CAD build for the part. Positions are in the model's coordinates, mm. Face numbers are marked on the shaded views. A direction names the side the tool comes from. Round coordinates to 2 decimals unless told otherwise and drop trailing zeros. Loops run counter-clockwise (first coordinate to the right, second up) from the corner with the lowest first, then second, coordinate; pieces in that order, holes last.
from build123d import *

# Parameters (mm, degrees)
SKETCH_1_R          = 3.1
EXTRUDE_1_DEPTH     = 5.7
SKETCH_2_R          = 2
EXTRUDE_2_DEPTH     = 7
SKETCH_3_R          = 1.25
EXTRUDE_3_DEPTH     = 6
CHAMFER_1_SIZE      = 0.2535
CHAMFER_2_SIZE      = 0.5
SKETCH_5_W          = 1.1
SKETCH_5_H          = 7
CUT_EXTRUDE_1_DEPTH = 1.2


with BuildPart() as part:
    # Эскиз1 → Бобышка-Вытянуть1 (new body)
    with BuildSketch(Plane.XY):
        Circle(SKETCH_1_R)
    extrude(amount=EXTRUDE_1_DEPTH)

    # Эскиз2 → Бобышка-Вытянуть2 (add)
    with BuildSketch(Plane(origin=(0, 0, 0), x_dir=(-1, 0, 0), z_dir=(0, 0, -1))):
        Circle(SKETCH_2_R)
    extrude(amount=EXTRUDE_2_DEPTH)

    # Эскиз3 → Бобышка-Вытянуть3 (add)
    with BuildSketch(Plane(origin=(0, 0, -7), x_dir=(-1, 0, 0), z_dir=(0, 0, -1))):
        Circle(SKETCH_3_R)
    extrude(amount=EXTRUDE_3_DEPTH)

    # Фаска1
    chamfer_1_edges = [part.edges().sort_by_distance(p)[0] for p in [
        (1.25, 0, -13),
    ]]
    chamfer(chamfer_1_edges, length=CHAMFER_1_SIZE)

    # Фаска2
    chamfer_2_edges = [part.edges().sort_by_distance(p)[0] for p in [
        (-3.1, 0, 5.7),
    ]]
    chamfer(chamfer_2_edges, length=CHAMFER_2_SIZE)

    # Эскиз5 → Вырез-Вытянуть1 (cut)
    with BuildSketch(Plane.XY.offset(5.7)):
        Rectangle(SKETCH_5_W, SKETCH_5_H)
    extrude(amount=-CUT_EXTRUDE_1_DEPTH, mode=Mode.SUBTRACT)


solid = part.part
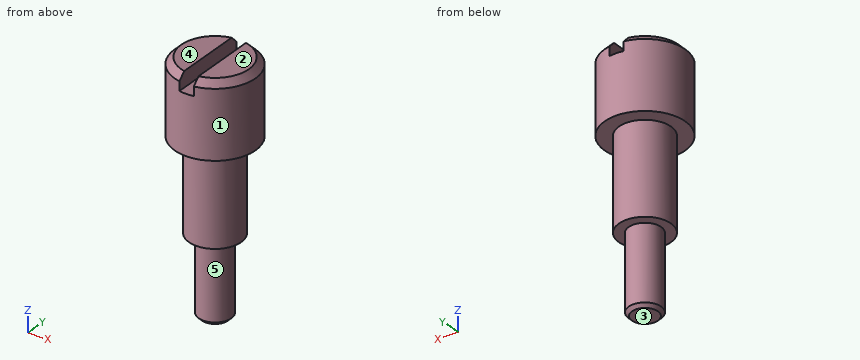
Item 1: Cut at C-C (z = -3.5). List the corners of the cut face in (x, y), plus the area to 3 significant figures.
Verdict:
outline: circle Ø4 at (0, 0)
area: 12.6 mm2
Item 2: Wall check: L1, parallel to Z at x = -0.75, y = 2; L2, parallel to Z at x = -0.5, y = 1.75; L3, parallel to X at y = -0.75, z = -7.5. Give the ranges that are in metal, low to high.
Verdict:
L1: z = 0 to 5.7
L2: z = -7 to 4.5
L3: x = -1 to 1
Item 3: Cut at B-B (x = 0). List the corners of the cut face in (y, z), plus the area to 3 significant figures.
Verdict:
outline: (-3.1, 0) - (-2, 0) - (-2, -7) - (-1.25, -7) - (-1.25, -12.75) - (-1, -13) - (1, -13) - (1.25, -12.75) - (1.25, -7) - (2, -7) - (2, 0) - (3.1, 0) - (3.1, 4.5) - (-3.1, 4.5) - close
area: 70.8 mm2
Item 4: Mould opens along Z. For the marked faces 1, 2 and 3 say: released by +Z, released by -Z, zero draft, split by the parting line, or undercut.
Verdict:
face 1: zero draft
face 2: released by +Z
face 3: released by -Z
Item 5: 3-axis set-ups, long thin cutter, end or side, ignore diameter. For the marked faces 4 and 5: which of +Z, -Z, +X, -X, +Y, -Y reach the whole face in a straight line?
Verdict:
face 4: +Z, +X, -X, +Y, -Y
face 5: -Z
Item 6: Cut at A-A (y = 0). List the corners of the cut face in (x, z).
Verdict:
outline: (-3.1, 0) - (-2, 0) - (-2, -7) - (-1.25, -7) - (-1.25, -12.75) - (-1, -13) - (1, -13) - (1.25, -12.75) - (1.25, -7) - (2, -7) - (2, 0) - (3.1, 0) - (3.1, 5.2) - (2.6, 5.7) - (0.55, 5.7) - (0.55, 4.5) - (-0.55, 4.5) - (-0.55, 5.7) - (-2.6, 5.7) - (-3.1, 5.2) - close
Item 7: Flat gauge pins, fed straight in: P1, Ø0.6, axis at x = 0, y = 0, coming from the +Z side; P2, Ø3, axis at x = -1.5, z = -3, coming from the +Y side; P3, Ø2, axis at x = 1.5, y = -2.5, coming from the -Z side. Where does each tip first touch, or does it go through?
Verdict:
P1: stops at z = 4.5
P2: stops at y = 2
P3: stops at z = -7
